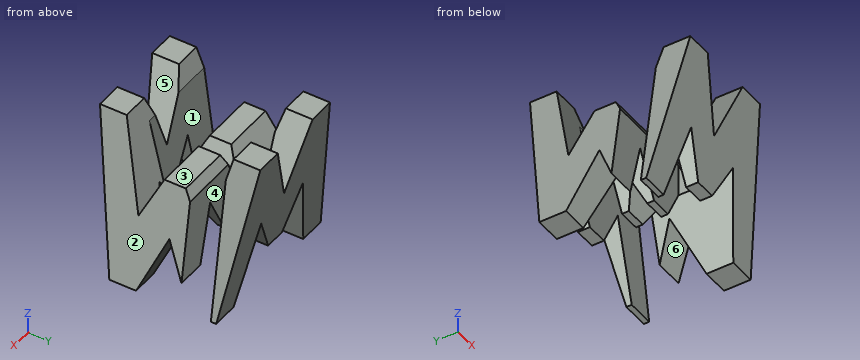
```python
from build123d import *

# Parameters (mm, degrees)
F0_W      = 38.1
F0_H      = 38.1
F1_DEPTH  = 38.1
F6_DEPTH  = 38.1
F8_DEPTH  = 38.1
F9_W      = 25.4
F9_H      = 7.62
F10_DEPTH = 38.1


with BuildPart() as f1:
    # F0 (on Front) → F1 (new body)
    with BuildSketch(Plane.XZ):
        with Locations((19.05, 19.05)):
            Rectangle(F0_W, F0_H)
    extrude(amount=F1_DEPTH)

    # F5 (on offset) → F6 (cut)
    with BuildSketch(Plane.YZ.offset(38.1)):
        Polygon((-6.35, 38.1), (-31.75, 38.1), (-26.67, 16.848067), (-21.59, 27.249678), (-16.51, 27.249678), (-11.43, 16.848067), align=None)
        Polygon((-31.75, 0), (-38.1, 38.1), (-38.1, 0), align=None)
        Polygon((-19.05, 14.549678), (-25.4, 0), (-12.7, 0), align=None)
        Polygon((0, 0), (0, 38.1), (-6.35, 0), align=None)
    extrude(amount=-F6_DEPTH, mode=Mode.SUBTRACT)

    # F7 (on offset) → F8 (cut)
    with BuildSketch(Plane.XZ.offset(38.1)):
        Polygon((25.4, 38.1), (12.7, 38.1), (19.05, 22.225), align=None)
        Polygon((0, 38.1), (0, 0), (6.35, 38.1), align=None)
        Polygon((31.75, 38.1), (38.1, 0), (38.1, 38.1), align=None)
        Polygon((11.43, 19.493997), (6.35, 0), (31.75, 0), (26.67, 19.493997), (21.59, 9.525), (16.51, 9.525), align=None)
    extrude(amount=-F8_DEPTH, mode=Mode.SUBTRACT)

    # F9 (on offset) → F10 (cut)
    with BuildSketch(Plane.XY.offset(38.1)):
        with Locations((25.4, -11.43)):
            Rectangle(F9_W, F9_H)
        with Locations((12.7, -26.67)):
            Rectangle(F9_W, F9_H)
    extrude(amount=-F10_DEPTH, mode=Mode.SUBTRACT)


solid = f1.part
```
Design review of the part built by this model. Coordinates are the model's own, in mm. Face numbers are marked on the shaded views. A direction names the side the tool comes from. Coordinates: 2 decimals unless noted, no trailing zeros. Loops run counter-clockwise (first coordinate to the right, second up) from the corner with the lowest first, then second, coordinate; pieces in that order, holes last. Notation, with made-up numbers: (-8.75, 42.25) - (41.25, 42.25) arc R23 cw to (41.25, 81.25) - close; hole circle Ø3 at (66.25, 55.25). An arc over 180 degrees is marked (long way). Use CSV: the item, a comma, the result in double quotes. Start each with the question number.
1) Consider section A-A on z = 31.5. Write out the cut boundary in (x, y).
2) For pin 1 Ø3 at (x, y) = (19.5, -5.5) entering from -Z (3 decimals); pin 2 Ø1.5 at (x, z) = (32.5, 20.5) entering from -Y; pin 3 Ø5 at (x, z) = (23, 8) entering from -Y; pin 4 Ø5 at (y, z) = (-15, 30) entering from +X, all flat-tipped, find the tip position at first contact; note any pin that passes through.
3) Consider section C-C on y = -24.5. Write out the cut boundary in (x, z), then the cut area to 3 significant figures.
4) The part is to be moulded in two halves that separate along Y. For the marked faces 1, 2 and 3, say which applies: +Y half, -Y half, draft (parallel to the pull), parting line (faces both ways), or undercut.
5) Consider section B-B on x = 15.5. Write out the cut boundary in (y, z), then the cut area to 3 significant figures.
6) Tool access review of the marked faces 4, 5 and 6: name each direction out of +Z, -Z, +X, -X, +Y, -Y from which nothing blocks a thin tool from reaching the whole face with its end or side.
7) Wall thickness on L1, parallel to X at y = -22, z = 19; L2, parallel to Y at x = 13.5, z = 22.5; L3, parallel to Y at x = 18.5, z = 18.5: over which ranges is each line inside the solid? List them lowest first. Write a range as from..to.
8) Consider section D-D on z = 8.5. Write out the cut boundary in (x, y), then the cut area to 3 significant figures.
Geometry says:
1,outline,"(5.25, -37) - (15.34, -37) - (15.34, -30.48) - (5.25, -30.48) - close; (5.25, -7.93) - (12.7, -7.93) - (12.7, -7.62) - (15.34, -7.62) - (15.34, -1.1) - (5.25, -1.1) - close; (22.76, -37) - (32.85, -37) - (32.85, -30.17) - (25.4, -30.17) - (25.4, -30.48) - (22.76, -30.48) - close; (22.76, -7.62) - (32.85, -7.62) - (32.85, -1.1) - (22.76, -1.1) - close"
2,pin 1,"z = 9.525"
2,pin 2,"y = -35.29"
2,pin 3,"y = -33.46"
2,pin 4,"through"
3,outline,"(25.4, 17) - (26.67, 19.49) - (31.21, 2.06) - (37.76, 2.06) - (34.55, 21.29) - (25.4, 21.29) - close"
3,area,"147 mm^2"
4,face 1,"undercut"
4,face 2,"draft"
4,face 3,"undercut"
5,outline,"(-36.93, 31.1) - (-33.67, 11.51) - (-30.48, 11.51) - (-30.48, 31.1) - close; (-22.86, 11.51) - (-20.38, 11.51) - (-19.05, 14.55) - (-17.72, 11.51) - (-15.24, 11.51) - (-15.24, 24.65) - (-16.51, 27.25) - (-21.59, 27.25) - (-22.86, 24.65) - close; (-7.62, 11.51) - (-4.43, 11.51) - (-1.17, 31.1) - (-7.62, 31.1) - close"
5,area,"302 mm^2"
6,face 4,"+Z, -Z, +X"
6,face 5,"+Z, +Y, -Y"
6,face 6,"-Z, +X, -X"
7,L1,"3.17..11.3, 11.68..26.42, 26.8..34.93"
7,L2,"-35.5..-30.48, -22.86..-15.24, -7.62..-2.6"
7,L3,"-34.83..-30.48, -22.86..-15.24, -7.62..-3.27"
8,outline,"(1.42, -33.17) - (8.57, -33.17) - (8.57, -30.48) - (1.42, -30.48) - close; (1.42, -22.86) - (8.57, -22.86) - (8.57, -21.69) - (1.42, -21.69) - close; (1.42, -16.41) - (8.57, -16.41) - (8.57, -4.93) - (1.42, -4.93) - close; (29.53, -33.17) - (36.68, -33.17) - (36.68, -21.69) - (29.53, -21.69) - close; (29.53, -16.41) - (36.68, -16.41) - (36.68, -15.24) - (29.53, -15.24) - close; (29.53, -7.62) - (36.68, -7.62) - (36.68, -4.93) - (29.53, -4.93) - close"
8,area,"219 mm^2"
